```python
from build123d import *


with BuildPart() as part:
    # Sketch1 → Revolve1 (revolve)
    with BuildSketch(Plane.XY):
        with BuildLine():
            Line((50, 0), (50, 20))
            ThreePointArc((50, 20), (49.707106781, 20.707106781), (49, 21))
            Line((49, 21), (47.577350269, 21))
            ThreePointArc((47.577350269, 21), (47.077350269, 20.866025404), (46.711324865, 20.5))
            Line((46.711324865, 20.5), (44.690598923, 17))
            ThreePointArc((44.690598923, 17), (43.958548116, 16.267949192), (42.958548116, 16))
            Line((42.958548116, 16), (18.618802154, 16))
            ThreePointArc((18.618802154, 16), (17.618802154, 16.267949192), (16.886751346, 17))
            Line((16.886751346, 17), (14.288675135, 21.5))
            ThreePointArc((14.288675135, 21.5), (13.922649731, 21.866025404), (13.422649731, 22))
            Line((13.422649731, 22), (7, 22))
            Line((7, 22), (0, 15))
            Line((0, 15), (0, 0))
            Line((0, 0), (50, 0))
        make_face()
    revolve(axis=Axis((0, 0, 0), (1, 0, 0)))


solid = part.part
```
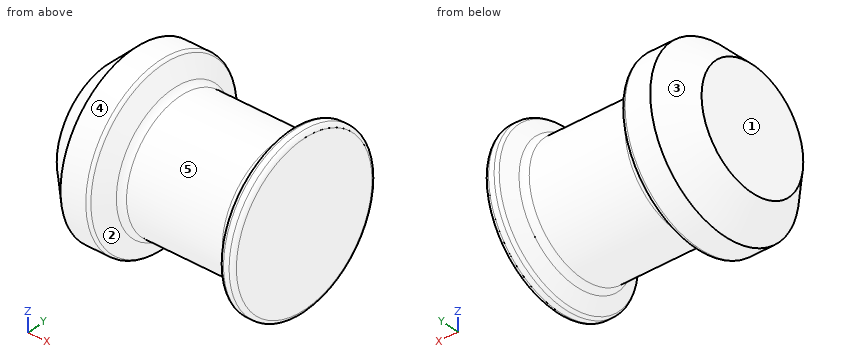
Can you work these out from the model? Positions are in its coordinate system, mm. Face numbers are marked on the shaded views. A direction names the side the tool comes from. Give positions to 0.01 mm unless a question says otherwise; leave off trailing zeros. Write each loop counter-clockwise with the first axis right and the second up, starting at its lowest first coordinate (ties: lowest second). Pieces come first, ordered by that corner, then holes. Notation, with made-up numbers: (-17.5, 0.5) -> (11.5, 0.5) arc R23 cw to (11.5, 23.5) -> close; hole circle Ø2 at (29.5, 54). An arc over 180 degrees is marked (long way). One line per item, written item: value.
Q1. Imagine slicing it at C-C on x = 12. Please give me the cut outline in (y, z), and give its area (3 significant figures).
Results found:
outline: circle Ø44 at (0, 0)
area: 1,520 mm^2
Q2. For P1, Ø4, axis at x = 13, y = 11, coming from the -Z side; P2, Ø1.5, axis at x = 6, y = 9.5, coming from the -Z side; P3, Ø12, axis at x = 30, z = -11.5, coming from the +Y side (3 decimals); P4, Ø8, axis at y = 5.5, z = 3.5, coming from the -X side, each with a flat end and sliding along its axis, tell me the tip position at first contact or that it passes through.
Results found:
P1: stops at z = -20.07
P2: stops at z = -19.64
P3: stops at y = 15.025
P4: stops at x = 0
Q3. Imagine slicing it at A-A on y = 0. Please give me the cut outline in (x, z), and give its area (3 significant figures).
Results found:
outline: (0, -15) -> (7, -22) -> (13.42, -22) arc R1 ccw to (14.29, -21.5) -> (16.89, -17) arc R2 cw to (18.62, -16) -> (42.96, -16) arc R2 cw to (44.69, -17) -> (46.71, -20.5) arc R1 ccw to (47.58, -21) -> (49, -21) arc R1 ccw to (50, -20) -> (50, 20) arc R1 ccw to (49, 21) -> (47.58, 21) arc R1 ccw to (46.71, 20.5) -> (44.69, 17) arc R2 cw to (42.96, 16) -> (18.62, 16) arc R2 cw to (16.89, 17) -> (14.29, 21.5) arc R1 ccw to (13.42, 22) -> (7, 22) -> (0, 15) -> close
area: 1,780 mm^2
Q4. We'd pull the mould along X, two halves only. Please class the marked faces 3, 4 and 5: +X half, -X half, draft (parallel to the pull), parting line (faces both ways), or undercut.
Results found:
face 3: -X half
face 4: draft
face 5: undercut
Q5. Imagine slicing it at D-D on x = 30. Please give me the cut outline in (y, z).
Results found:
outline: circle Ø32 at (0, 0)
Q6. Which directions (+Z, -Z, +X, -X, +Y, -Y) give clear straight access to the entire face, cutting with the end or side of a thin tool? Please do the marked faces 1 and 2.
Results found:
face 1: +Z, -Z, -X, +Y, -Y
face 2: none
Q7. Please list where these lines run through material, in increasing order: line 1 (X direction, y = 12, z = -16); line 2 (X direction, y = -4.5, z = 20); line 3 (Y direction, x = 10.5, z = -3). Write a range as [from, to].
Results found:
line 1: x = [5, 15.15], [46.42, 50]
line 2: x = [5.5, 14.87], [46.71, 49.87]
line 3: y = [-21.79, 21.79]
